Source: three-view drawing plus pictorial views. Frame: mm from the lowest corner of the part. Give positions to 0.01 mm unless a question says otherwise; leave off trailing zeros. Loops run counter-clockwise (first coordinate to the right, second up) from the corner with the lowest first, then second, coordinate; pieces in that order, holes last.
1. First-contact query: P1, Ø2.5, axis at x = 88.5, z = 5, coming from the +Y side; P2, Ø2, axis at y = 115.5, z = 3.5, coming from the -X side; P3, Ø2.5, axis at y = 93, z = 5, coming from the -X side. Flat tips, straight axial feed; report the tip coordinate or a pass-through.
2. Section B-B, the plane x = 161.5. Output: boundary loops of the cut face in (y, z) (3 decimals), then the cut area to 3 significant figures.
3. Material intervals for line 1 along Y through (x, z) = (143, 1.5); line 2 along X through (y, z) = (79, 3); line 3 along X through (y, z) = (37.5, 6), sorted ascending.
4. Section A-A, the plane y = 79. Output: boundary loops of the cut face in (x, z) (3 decimals).
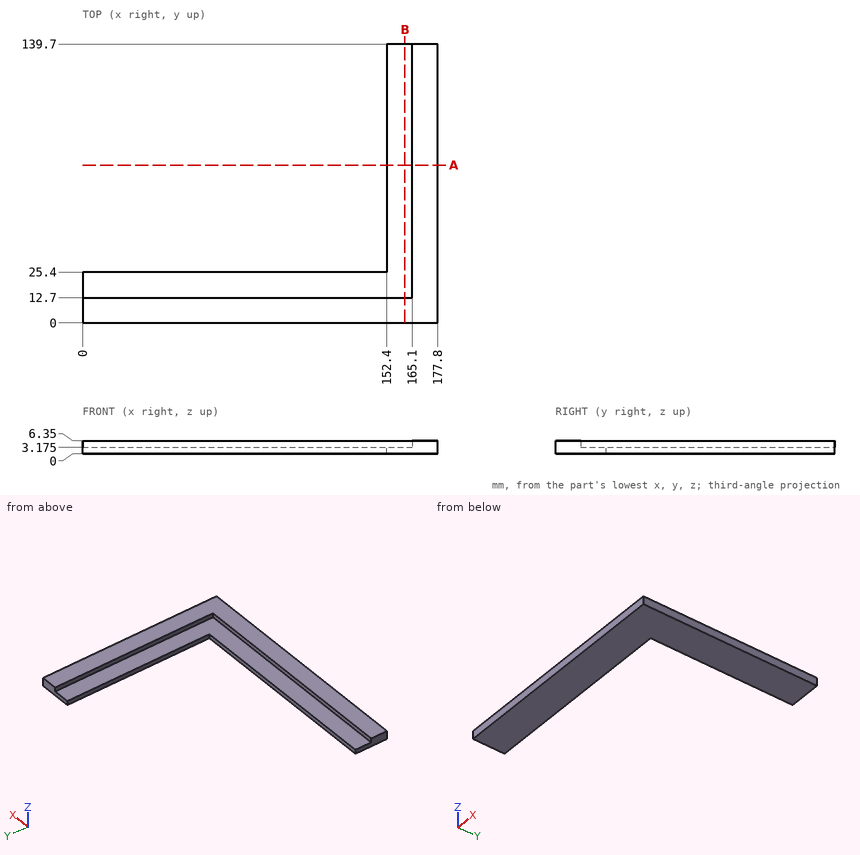
Answers below:
1. P1: stops at y = 12.7
1. P2: stops at x = 152.4
1. P3: stops at x = 165.1
2. outline: (0, 0) - (139.7, 0) - (139.7, 3.175) - (12.7, 3.175) - (12.7, 6.35) - (0, 6.35) - close
2. area: 484 mm2
3. line 1: y = 0 to 25.4
3. line 2: x = 152.4 to 177.8
3. line 3: x = 165.1 to 177.8
4. outline: (152.4, 0) - (177.8, 0) - (177.8, 6.35) - (165.1, 6.35) - (165.1, 3.175) - (152.4, 3.175) - close
